The model under review builds one solid part; all positions refer to its coordinate system, in mm. Face numbers are marked on the shaded views. A direction names the side the tool comes from. Coordinates: 2 decimals unless noted, no trailing zeros. Write each loop counter-clockwise with the first axis right and the second up, starting at its lowest first coordinate (ties: lowest second). Pieces come first, ordered by that corner, then holes. Notation, with made-up numbers: (36.5, -16) - (57.5, -16) arc R14 cw to (57.5, -9) - close; hole circle Ø6 at (31.25, 6.25). An arc over 180 degrees is marked (long way). Return JSON: item names as keys, results as strings. Group by question number.
(1) We need section A-A on z = 6. State the section outline as (x, y) points.
(2) Tool access review of the marked faces 4, 5 and 6: name each direction out of +Z, -Z, +X, -X, +Y, -Y from which nothing blocks a thin tool from reaching the whole face with its end or side.
(3) We need section B-B on x = 0. State the section outline as (y, z) points, then the cut area to 3 significant figures.
(4) We need section C-C on y = -1.5. State the section outline as (x, z) points, then the cut area to 3 significant figures.
(5) To check wall thickness, follow L1, parallel to X at y = 4, z = 17; L2, parallel to Y at x = 8.4, z = 13; L3, parallel to Y at x = -9, z = 13. State the ranges of each line that lie inside material, in increasing order. Write a range as from..to.
(6) We need section D-D on z = 12. State the section outline as (x, y) points, then the cut area to 3 significant figures.
(7) For pin 1 Ø6 at (x, z) = (2.5, 19) entering from +Y; pin 2 Ø6 at (x, y) = (3.5, -4) entering from -Z; pin 3 Ø10 at (y, z) = (3.5, 11) entering from -X; pin 4 Ø0.5 at (y, z) = (-9.5, -1) entering from +X, all flat-tipped, find the tip position at first contact; note any pin that passes through.
(8) Draft analysis for pull direction Y (two halves, no side actions). For the marked faces 1, 2 and 3, state which applies: released by +Y, released by -Y, zero draft, split by the parting line, or undercut.
```python
from build123d import *

# Parameters (mm, degrees)
SKETCH_1_W          = 20
SKETCH_1_H          = 20
EXTRUDE_1_DEPTH     = 3
SKETCH_2_W          = 3
SKETCH_2_H          = 20
EXTRUDE_2_DEPTH     = 20
CUT_EXTRUDE_START   = -20
CUT_EXTRUDE_2_DEPTH = 20
SKETCH_4_R          = 2
CUT_EXTRUDE_3_DEPTH = 33.078029865
SKETCH_5_R          = 5
CUT_EXTRUDE_4_DEPTH = 2
SKETCH_6_R          = 3
CUT_EXTRUDE_5_DEPTH = 25.494897428
SKETCH_7_W          = 8.2
SKETCH_7_H          = 1
EXTRUDE_3_DEPTH     = 2


# Read off the part's stored shape, not the designer's step: 切除-拉伸2
with BuildPart() as part:
    # 草图1 → 凸台-拉伸1 (new body)
    with BuildSketch(Plane.XY):
        Rectangle(SKETCH_1_W, SKETCH_1_H)
    extrude(amount=EXTRUDE_1_DEPTH)

    # 草图2 → 凸台-拉伸2 (add)
    with BuildSketch(Plane.XY.offset(3)):
        with Locations((-8.5, 0)):
            Rectangle(SKETCH_2_W, SKETCH_2_H)
        with Locations((8.5, 0)):
            Rectangle(SKETCH_2_W, SKETCH_2_H)
    extrude(amount=EXTRUDE_2_DEPTH)

    # 切除-拉伸2 outline → 切除-拉伸2 (cut)
    with BuildSketch(Plane.ZY.offset(10).offset(CUT_EXTRUDE_START)):
        with BuildLine():
            Line((23, 10), (13, 10))
            ThreePointArc((13, 10), (20.071067812, 7.071067812), (23, 0))
            Line((23, 0), (23, 10))
        make_face()
        with BuildLine():
            Line((23, -10), (23, 0))
            ThreePointArc((23, 0), (20.071067812, -7.071067812), (13, -10))
            Line((13, -10), (23, -10))
        make_face()
    extrude(amount=CUT_EXTRUDE_2_DEPTH, mode=Mode.SUBTRACT)

    # 草图4 → 切除-拉伸3 (cut, through all)
    with BuildSketch(Plane.ZY.offset(10)):
        with Locations((13, 0)):
            Circle(SKETCH_4_R)
    extrude(amount=-CUT_EXTRUDE_3_DEPTH, mode=Mode.SUBTRACT)

    # 草图5 → 切除-拉伸4 (cut)
    with BuildSketch(Plane.ZY.offset(10)):
        with Locations((13, 0)):
            Circle(SKETCH_5_R)
    extrude(amount=-CUT_EXTRUDE_4_DEPTH, mode=Mode.SUBTRACT)

    # 草图6 → 切除-拉伸5 (cut, through all)
    with BuildSketch(Plane.XY.offset(3)):
        Circle(SKETCH_6_R)
    extrude(amount=-CUT_EXTRUDE_5_DEPTH, mode=Mode.SUBTRACT)

    # 草图7 → 凸台-拉伸3 (add)
    with BuildSketch(Plane(origin=(0, 0, 0), x_dir=(-1, 0, 0), z_dir=(0, 0, -1))):
        with Locations((0, 9.5)):
            Rectangle(SKETCH_7_W, SKETCH_7_H)
        with Locations((0, -9.5)):
            Rectangle(SKETCH_7_W, SKETCH_7_H)
    extrude(amount=EXTRUDE_3_DEPTH)


solid = part.part
```
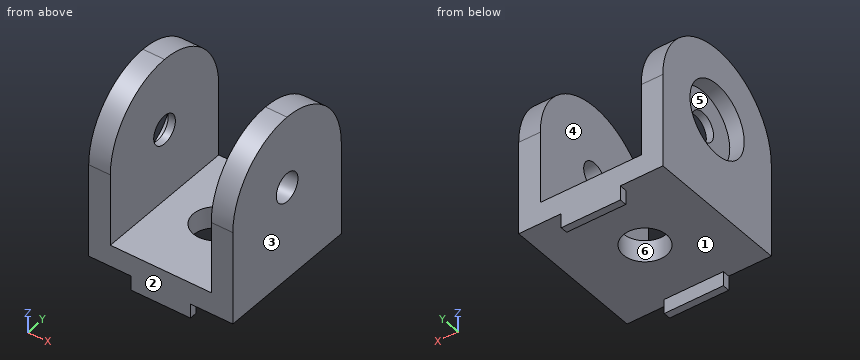
Ans:
{
 "1": {"outline": "(-10, -10) - (-7, -10) - (-7, 10) - (-10, 10) - close; (7, -10) - (10, -10) - (10, 10) - (7, 10) - close"},
 "2": {"face 4": "+Z, +Y, -Y", "face 5": "-X", "face 6": "+Z, -Z"},
 "3": {"outline": "(-10, -2) - (-9, -2) - (-9, 0) - (-3, 0) - (-3, 3) - (-10, 3) - close; (3, 0) - (9, 0) - (9, -2) - (10, -2) - (10, 3) - (3, 3) - close", "area": "46.0 mm²"},
 "4": {"outline": "(-10, 0) - (-2.6, 0) - (-2.6, 3) - (-7, 3) - (-7, 11.68) - (-8, 11.68) - (-8, 8.23) - (-10, 8.23) - close; (-10, 17.77) - (-8, 17.77) - (-8, 14.32) - (-7, 14.32) - (-7, 22.89) - (-10, 22.89) - close; (2.6, 0) - (10, 0) - (10, 11.68) - (7, 11.68) - (7, 3) - (2.6, 3) - close; (7, 14.32) - (10, 14.32) - (10, 22.89) - (7, 22.89) - close", "area": "134 mm²"},
 "5": {"L1": "-10..-7, 7..10", "L2": "-10..-2, 2..10", "L3": "-10..-5, 5..10"},
 "6": {"outline": "(-10, -10) - (-7, -10) - (-7, -1.73) - (-8, -1.73) - (-8, -4.9) - (-10, -4.9) - close; (-10, 4.9) - (-8, 4.9) - (-8, 1.73) - (-7, 1.73) - (-7, 10) - (-10, 10) - close; (7, -10) - (10, -10) - (10, -1.73) - (7, -1.73) - close; (7, 1.73) - (10, 1.73) - (10, 10) - (7, 10) - close", "area": "86.5 mm²"},
 "7": {"pin 1": "through", "pin 2": "z = 0", "pin 3": "x = -10", "pin 4": "x = 4.1"},
 "8": {"face 1": "undercut", "face 2": "released by -Y", "face 3": "zero draft"}
}
